```python
from build123d import *

# Parameters (mm, degrees)
F0_W        = 50.8
F0_H        = 34.9398194141
F1_DEPTH    = 25.4
F0_W_2      = 9.2941272077
F0_H_2      = 22.9654247603
F3_T1_DEPTH = 129.872769086


# Not quite as in the source:
# - a fillet or chamfer that OpenCascade refuses, or shapes differently, is made with other operations: its cross-section is extruded or revolved along the edge and cut away or added


with BuildPart() as f1:
    # F0 (on Top) → F1 (new body)
    with BuildSketch(Plane.XY):
        with Locations((34.6941272077, 40.4353344673)):
            Rectangle(F0_W, F0_H)
    extrude(amount=F1_DEPTH)

    # F0 (on Top) → F2 (revolve)
    with BuildSketch(Plane.XY):
        with Locations((4.6470636039, 11.4827123801)):
            Rectangle(F0_W_2, F0_H_2)
    revolve(axis=Axis((9.2941272077, 11.4827123801, 0), (0, 1, 0)))

    # F3: fillet of radius 41.0850864045 on 1 edges, made by hand

    # F3_s2 → F3_t1 (cut)
    with BuildSketch(Plane.XZ.offset(-152.8381938463)):
        with BuildLine():
            ThreePointArc((9.2941272077, 0), (24.4247897604, 18.4646387412), (47.2673070765, 25.4))
            Line((47.2673070765, 25.4), (9.2941272077, 25.4))
            Line((9.2941272077, 25.4), (9.2941272077, 0))
        make_face()
    extrude(amount=F3_T1_DEPTH, mode=Mode.SUBTRACT)


solid = f1.part
```
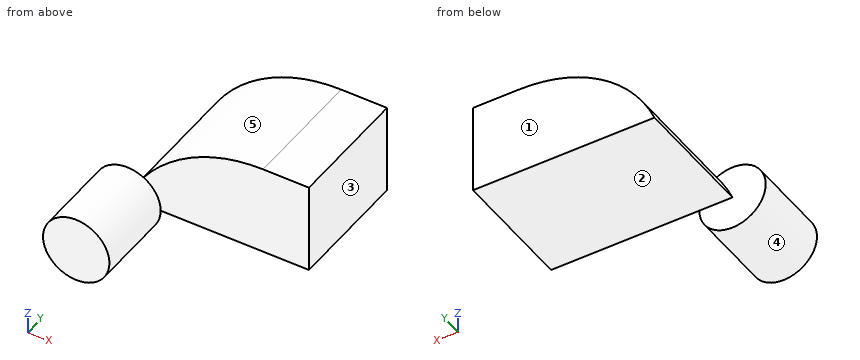
Here's how the part is built. I have some questions about the finished solid (model axes, mm). Face numbers are marked on the shaded views. A direction names the side the tool comes from. Coordinates: 2 decimals unless noted, no trailing zeros. Write each loop counter-clockwise with the first axis right and the second up, starting at its lowest first coordinate (ties: lowest second). Pieces come first, ordered by that corner, then holes. Notation, with made-up numbers: (70, 14) - (106, 14) arc R20 ccw to (106, 39) - close; hole circle Ø11 at (4.5, -34). An arc over 180 degrees is marked (long way). One line per item, written item: value.
1) Suppose I cut it at A-A on y = 34. Write out the boundary of the cut face in (x, z).
Model answer:
outline: (9.29, 0) - (60.09, 0) - (60.09, 25.4) - (47.27, 25.4) arc R41.09 ccw to start
2) I'm going to push flat-ended pins straight in: P1, Ø10.5, axis at x = 42.5, y = 36.5, coming from the -Z side; P2, Ø5.5, axis at x = 5.5, z = 2, coming from the +Y side; P3, Ø12, axis at x = 24.5, y = 27, coming from the +Z side. Where does each tip first touch, or does it pass through?
Model answer:
P1: stops at z = 0
P2: stops at y = 22.97
P3: stops at z = 21.82
3) Suppose I cut it at B-B on x = 42. Write out the boundary of the cut face in (y, z), and give its area (3 significant figures).
Model answer:
outline: (22.97, 0) - (57.91, 0) - (57.91, 25.06) - (22.97, 25.06) - close
area: 876 mm²
4) On a 3-axis mill with a long thin cutter (end or side, diameter ignored), from which of +Z, -Z, +X, -X, +Y, -Y can I reach the whole of each face in a straight line? I mean the marked faces 1, 2, 3, 4 and 5. Say none if no direction works.
Model answer:
face 1: +Z, -Z, +X, -X, +Y
face 2: -Z, +X, -X, +Y
face 3: +Z, -Z, +X, +Y, -Y
face 4: -Y
face 5: +Z, -X, +Y
5) I need wall thicknesses on line 1 along Y through (x, z) = (31.5, 2); line 2 along Y through (x, z) = (5, -4); line 3 along Z through (x, y) = (13, 38.5). Which ranges of each line are inside material? Lowest first, please.
Model answer:
line 1: y = 22.97 to 57.91
line 2: y = 0 to 22.97
line 3: z = 0 to 6.98
